Verification items for the finished model (mm, model axes). Face numbers are marked on the shaded views. A direction names the side the tool comes from. Round coordinates to 2 decimals unless told otherwise and drop trailing zeros. Order: outer loops, then holes, each group sorted by start corner. A loop starts at its lowest first (then second) coordinate and runs counter-clockwise, first axis right, second up. Notation, with made-up numbers: M 64.5,-26.75 L 108.5,-26.75 A14 ccw 108.5,0.25 Z; hole C -28.5,23 d10. An arc over 180 degrees is marked long. Answer as a JSON object with one key per item and string values. Group by question number.
Autodesk Inventor part; units mm, degrees
ref_plane "Work Plane1" through (-70, 0, 0) normal (1, 0, 0) x (0, 1, 0)
ref_plane "XZ Plane" through (0, 0, 0) normal (0, 1, 0) x (-1, 0, 0)
ref_plane "XY Plane" through (0, 0, 0) normal (0, 0, 1) x (1, 0, 0)
sketch "Sketch1" plane through (0, 0, 0) normal (0, 1, 0) x (-1, 0, 0)
  circle A0 centre (0, 0) radius 112.5
  circle A1 centre (0, 0) radius 92.5 construction
  circle A2 centre (0, 0) radius 32.5
  circle A3 centre (92.5, 0) radius 10.25
  line L0 (157.5, 0) -> (-157.5, 0) construction
  circle A4 centre (65.4074, 65.4074) radius 10.25
  circle A5 centre (0, 92.5) radius 10.25
  circle A6 centre (-65.4074, 65.4074) radius 10.25
  circle A7 centre (-92.5, 0) radius 10.25
  circle A8 centre (-65.4074, -65.4074) radius 10.25
  circle A9 centre (0, -92.5) radius 10.25
  circle A10 centre (65.4074, -65.4074) radius 10.25
  dimension "d1" = 185
  dimension "d0" = 225
  dimension "d2" = 65
  dimension "d3" = 20.5
  dimension "d6" = 360
extrude "Extrusion1" add sketch "Sketch1" against normal blind 25
sketch "Sketch2" plane through (0, 0, 0) normal (0, 0, 1) x (1, 0, 0)
  line L0 (-112.5, -25) -> (112.5, -25)
  line L1 (0, -25) -> (0, -85)
  line L2 (90, -175) -> (145, -175)
  arc A0 (0, -85) -> (90, -175) centre (90, -85) ccw
  line L3 (112.5, 0) -> (-112.5, 0)
  point P0 (0, 0)
  point P1 (0, -175)
  dimension "d13" = 145
  dimension "d14" = 90
  dimension "d27" = 175
sketch "Sketch3" plane through (0, -25, 0) normal (0, -1, 0) x (1, 0, 0)
  circle A0 centre (0, 0) radius 48.5
  circle A1 centre (0, 0) radius 32.5
  dimension "d15" = 97
sweep "Sweep1" add profiles "Sketch3" path "Sketch2" path curves L1 A0 L2
sketch "Sketch4" plane through (145, -175, 0) normal (1, 0, 0) x (0, 0, -1)
  circle A0 centre (0, 0) radius 32.5
  circle A1 centre (0, 0) radius 48.5 construction
  circle A2 centre (0, 0) radius 112.5
  circle A3 centre (0, 0) radius 92.5
  line L0 (0, 0) -> (0, 112.5) construction
  circle A4 centre (0, 92.5) radius 10.25
  circle A5 centre (-65.4074, 65.4074) radius 10.25
  circle A6 centre (-92.5, 0) radius 10.25
  circle A7 centre (-65.4074, -65.4074) radius 10.25
  circle A8 centre (0, -92.5) radius 10.25
  circle A9 centre (65.4074, -65.4074) radius 10.25
  circle A10 centre (92.5, 0) radius 10.25
  circle A11 centre (65.4074, 65.4074) radius 10.25
  point P0 (0, 175)
  dimension "d18" = 225
  dimension "d19" = 185
  dimension "d20" = 20.5
  dimension "d23" = 360
extrude "Extrusion2" add sketch "Sketch4" along normal blind 25 contours A2 | A10 A3 A9 A8 A7 A6 A5 A4 A11
ref_plane "Work Plane1" through (-70, 0, 0) normal (1, 0, 0) x (0, 1, 0)
sketch "Sketch6" plane through (-70, 0, 0) normal (1, 0, 0) x (0, 1, 0)
  line L0 (0, -112.5) -> (0, 112.5) construction
  circle A0 centre (-175, 0) radius 112.5 construction
  circle A1 centre (-175, 0) radius 48.5 construction
  line L1 (0, 0) -> (-287.5, 0) construction
  circle A2 centre (-175, 0) radius 25
  dimension "d29" = 175
  dimension "d30" = 50
extrude "Extrusion3" add sketch "Sketch6" along normal up to next
hole "Hole1" at (-70, -175, 0) direction (1, 0, 0) diameter 20 end through all counterbore diameter 24 counterbore depth 28
properties part number "LE-2.3"
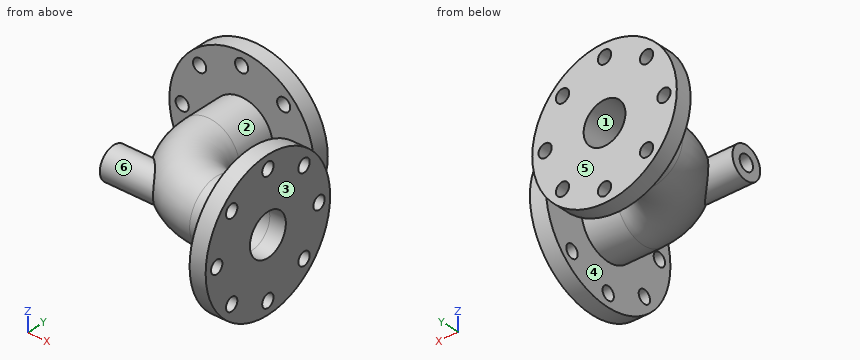
Q1. Cross-section at B-B, the plane z = 92.5. Record the cut outline in (x, y).
Q2. Cross-section at C-C, the plane y = -267.5. Record the cut outline in (x, z), then the cut area to 3 significant figures.
Q3. Cross-section at D-D, the plane x = -92.5. Record the cut outline in (y, z), then the cut area to 3 significant figures.
Q4. Tool access check on the marked faces 1, 2 and 3. Record the directions out of +Z, -Z, +X, -X, +Y, -Y that give a thin tool (end or side, any length) a straight path to the whole face; none if there is none.
Q5. Thickness scan on line 1 (Y direction, x = 153, z = 0); line 2 (Y direction, x = 52, z = 10); line 3 (Y direction, x = 72.5, z = -3.5). Record the ranges inside material, lowest first. Write a range as from..to.
Q6. Release check for a two-part mould opening along Y. For the marked faces 4, 5 and 6 record: released by +Y, released by -Y, zero draft, split by the parting line, or undercut.
Q7. Cross-section at A-A, the plane x = -64. Record the cut outline in (y, z).
Q8. Gauge pin test, flat ends, axial feed: pin 1 Ø3 at (x, z) = (-48.5, 73.5) entering from -Y; pin 2 Ø4 at (y, z) = (-231.5, 76.5) entering from -X; pin 3 Ø16.5 at (x, z) = (92.5, 0) entering from -Y; pin 4 Ø23.5 at (y, z) = (-82.5, 0) entering from +X. Record the tip position at first contact, or that the pin passes through.
Conclusion:
{
 "1": {"outline": "M -64.03,-25 L -10.25,-25 L -10.25,0 L -64.03,0 Z; M 10.25,-25 L 64.03,-25 L 64.03,0 L 10.25,0 Z; M 145,-239.03 L 170,-239.03 L 170,-185.25 L 145,-185.25 Z; M 145,-164.75 L 170,-164.75 L 170,-110.97 L 145,-110.97 Z"},
 "2": {"outline": "M 145,-64.03 L 170,-64.03 L 170,-10.25 L 145,-10.25 Z; M 145,10.25 L 170,10.25 L 170,64.03 L 145,64.03 Z", "area": "2,690 mm2"},
 "3": {"outline": "M -25,-64.03 L 0,-64.03 L 0,-10.25 L -25,-10.25 Z; M -25,10.25 L 0,10.25 L 0,64.03 L -25,64.03 Z", "area": "2,690 mm2"},
 "4": {"face 1": "+Y", "face 2": "none", "face 3": "+Z, -Z, +X, +Y, -Y"},
 "5": {"line 1": "-287.5..-277.75, -257.25..-207.5, -142.5..-92.75, -72.25..-62.5", "line 2": "-217.1..-199.8, -130.23..-104.13, -25..0", "line 3": "-222.26..-206.05, -139.97..-122.77, -25..0"},
 "6": {"face 4": "zero draft", "face 5": "released by +Y", "face 6": "undercut"},
 "7": {"outline": "C -175,0 d50; M -25,-92.52 L 0,-92.52 L 0,-75.56 L -25,-75.56 Z; M -25,-55.25 L 0,-55.25 L 0,55.25 L -25,55.25 Z; M -25,75.56 L 0,75.56 L 0,92.52 L -25,92.52 Z; hole C -175,0 d24"},
 "8": {"pin 1": "y = -25", "pin 2": "x = 145", "pin 3": "y = -223.5", "pin 4": "x = 170"}
}
